from build123d import *

# Parameters (mm, degrees)
F3_D           = 1
F3_DEPTH       = 65
F3_CBORE_D     = 38.3
F3_CBORE_DEPTH = 65
F3_TIP         = 0.3004303095
F5_D           = 7
F5_DEPTH       = 37.401


# Not quite as in the source:
# - a feature names something its author has since deleted; it is built from what else it names


with BuildPart() as f1:
    # F0 (on Front) → F1 (revolve)
    with BuildSketch(Plane.XZ):
        Polygon((0, 23.1), (0, 0), (125, 0), (125, 36.5), (52, 36.5), (52, 37.4), (50, 37.4), (50, 36.5), (50, 20.1), (38, 20.1), (38, 23.1), align=None)
    revolve(axis=Axis((62.5, 0, 0), (-1, 0, 0)))

    # F3
    with Locations(Plane.YZ.offset(125)):
        with Locations((0, 0)):
            CounterBoreHole(F3_D / 2, F3_CBORE_D / 2, F3_CBORE_DEPTH, depth=F3_DEPTH)
            with Locations((0, 0, -(F3_DEPTH + F3_TIP / 2))):  # 118° drill point
                Cone(0, F3_D / 2, F3_TIP, mode=Mode.SUBTRACT)

    # F5 (through all, one way)
    with BuildSketch(Plane(origin=(0, 0, 0), x_dir=(1, 0, 0), z_dir=(0, 0, -1))):
        with Locations((92.5, 0)):
            Circle(F5_D / 2)
    extrude(amount=-F5_DEPTH, mode=Mode.SUBTRACT)


solid = f1.part
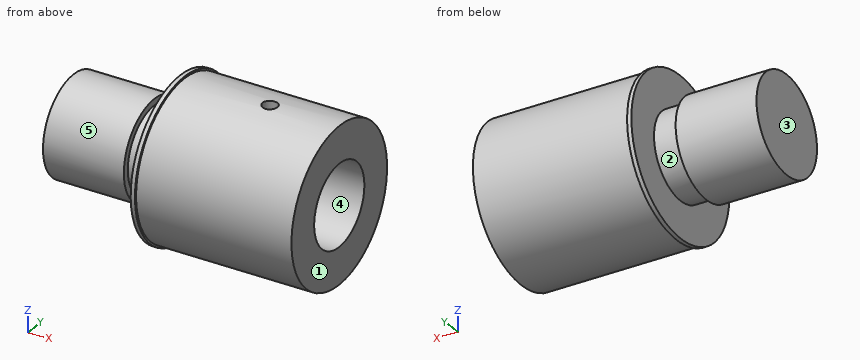
Geometry: final body of the model. Coordinates: model frame, mm. Face numbers are marked on the shaded views. A direction names the side the tool comes from. Coordinates: 2 decimals unless noted, no trailing zeros. Order: outer loops, then holes, each group sorted by start corner. A loop starts at its lowest first (then second) coordinate and runs counter-clockwise, first axis right, second up.
(1) Material intervals for probe 1 along X at (y, z) = (4.5, -22.5); probe 2 along X at (y, z) = (0, 29.5); probe 3 along X at (y, z) = (18.5, -17), sorted ascending.
(2) First-contact query: pin 1 (1.5 mm diameter, centred on y = -10.5, z = 3.5, fed in from +X); pin 2 (11 mm diameter, centred on x = 92.5, y = 0, fed in from -Z); pin 3 (12 mm diameter, centred on x = 77, y = 10, fed in from +Z); pin 4 (4 mm diameter, centred on y = 29, z = -29, fed in from +X). Flat tips, straight axial feed; report the tip coordinate or a pass-through.
(3) Access query for the marked faces 4 and 5. Directions: +Z, -Z, +X, -X, +Y, -Y. A direction counts if a zero-diameter tool reaches every point of the face in a straight line with its end or side. Return the directions, or none.
(4) Draft query along X for the marked faces 1, 2 and 3. Return one class per face: pulls with the +X half, pulls with the -X half, needs draft (parallel to the pull), parting line crosses it, or undercut.
(5) Section query A-A (z = 31). Return the cut outline in (x, y), plus the area to 3 significant figures.
(6) Section query C-C (y = -27). Return the cut outline in (x, z), plus the area to 3 significant figures.
(7) Section query D-D (z = -12). Return the cut outline in (x, y).
(8) Section query B-B (x = 106). Return the cut outline in (y, z).
Solution:
1. probe 1: x = 0 to 38, 50 to 125
1. probe 2: x = 50 to 89, 96 to 125
1. probe 3: x = 50 to 125
2. pin 1: stops at x = 60
2. pin 2: stops at z = -36.5
2. pin 3: stops at z = 36.28
2. pin 4: passes through
3. face 4: +X
3. face 5: -X
4. face 1: pulls with the +X half
4. face 2: undercut
4. face 3: pulls with the -X half
5. outline: (50, -20.92) - (52, -20.92) - (52, -19.27) - (125, -19.27) - (125, 19.27) - (52, 19.27) - (52, 20.92) - (50, 20.92) - close; hole circle Ø7 at (92.5, 0)
5. area: 2,860 mm2
6. outline: (50, -25.88) - (52, -25.88) - (52, -24.56) - (125, -24.56) - (125, 24.56) - (52, 24.56) - (52, 25.88) - (50, 25.88) - close
6. area: 3,690 mm2
7. outline: (0, -19.74) - (38, -19.74) - (38, -16.12) - (50, -16.12) - (50, -35.42) - (52, -35.42) - (52, -34.47) - (125, -34.47) - (125, -14.92) - (60, -14.92) - (60, 14.92) - (125, 14.92) - (125, 34.47) - (52, 34.47) - (52, 35.42) - (50, 35.42) - (50, 16.12) - (38, 16.12) - (38, 19.74) - (0, 19.74) - close
8. outline: circle Ø73 at (0, 0); hole circle Ø38.3 at (0, 0)
